Could you check a few things on this model? Use its own coordinates, in mm. Face numbers are marked on the shaded views. A direction names the side the tool comes from. Round coordinates to 2 decimals unless told otherwise and drop trailing zeros. Order: outer loops, then holes, each group sorted by start corner. A loop starts at its lowest first (then second) coordinate and runs counter-clockwise, first axis right, second up. Notation, with made-up numbers: (85, 39.5) - (97, 39.5) arc R6 ccw to (97, 50.5) - close; hole circle Ø4 at (35, 76). An arc over 180 degrees is marked (long way). Return JSON: item names as keys, results as strings. Group by question number.
from build123d import *

# Parameters (mm, degrees)
CROQUIS1_R              = 2.5
SALIENTE_EXTRUIR1_DEPTH = 36.2
CROQUIS2_OUTSIDE_W      = 14.376
CROQUIS2_OUTSIDE_H      = 14.376
CROQUIS2_OUTSIDE_W_2    = 5.186631864
CROQUIS2_OUTSIDE_H_2    = 3
CORTAR_EXTRUIR1_DEPTH   = 8
CROQUIS2_3_R            = 0.79375
CORTAR_EXTRUIR2_DEPTH   = 5
CROQUIS3_OUTSIDE_W      = 14.376
CROQUIS3_OUTSIDE_H      = 14.376
CORTAR_EXTRUIR3_DEPTH   = 8
CROQUIS4_R              = 0.79375
CORTAR_EXTRUIR4_DEPTH   = 5


with BuildPart() as part:
    # Croquis1 → Saliente-Extruir1 (new body)
    with BuildSketch(Plane(origin=(0, 0, 0), x_dir=(0, 0, -1), z_dir=(1, 0, 0))):
        Circle(CROQUIS1_R)
    extrude(amount=SALIENTE_EXTRUIR1_DEPTH)

    # Croquis2 outside → Cortar-Extruir1 (cut)
    with BuildSketch(Plane(origin=(36.2, 0, 0), x_dir=(0, 0, -1), z_dir=(1, 0, 0))):
        Rectangle(CROQUIS2_OUTSIDE_W, CROQUIS2_OUTSIDE_H)
        Rectangle(CROQUIS2_OUTSIDE_W_2, CROQUIS2_OUTSIDE_H_2, mode=Mode.SUBTRACT)
    extrude(amount=-CORTAR_EXTRUIR1_DEPTH, mode=Mode.SUBTRACT)

    # Croquis2_3 → Cortar-Extruir2 (cut)
    with BuildSketch(Plane(origin=(36.2, 0, 0), x_dir=(0, 0, -1), z_dir=(1, 0, 0))):
        Circle(CROQUIS2_3_R)
    extrude(amount=-CORTAR_EXTRUIR2_DEPTH, mode=Mode.SUBTRACT)

    # Croquis3 outside → Cortar-Extruir3 (cut)
    with BuildSketch(Plane(origin=(0, 0, 0), x_dir=(0, 0, -1), z_dir=(1, 0, 0))):
        Rectangle(CROQUIS3_OUTSIDE_W, CROQUIS3_OUTSIDE_H)
        with BuildLine():
            Line((2, 1.5), (-2, 1.5))
            ThreePointArc((-2, 1.5), (-2.5, 0), (-2, -1.5))
            Line((-2, -1.5), (2, -1.5))
            ThreePointArc((2, -1.5), (2.5, 0), (2, 1.5))
        make_face(mode=Mode.SUBTRACT)
    extrude(amount=CORTAR_EXTRUIR3_DEPTH, mode=Mode.SUBTRACT)

    # Croquis4 → Cortar-Extruir4 (cut)
    with BuildSketch(Plane.ZY):
        Circle(CROQUIS4_R)
    extrude(amount=-CORTAR_EXTRUIR4_DEPTH, mode=Mode.SUBTRACT)


solid = part.part
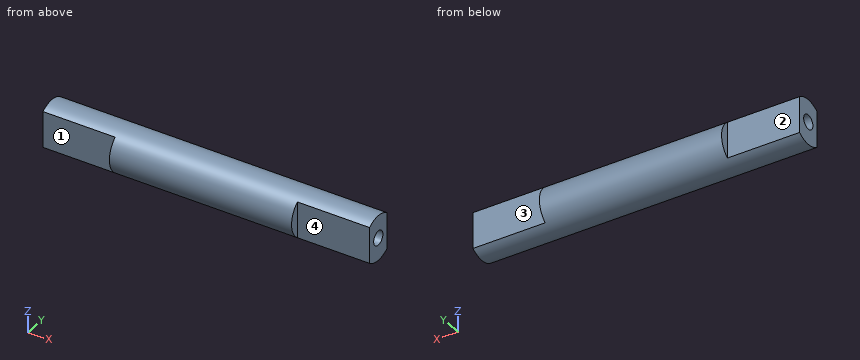
1) I want a section at C-C, the plane z = -1.5. List the corners of the cut face in (x, y) for me.
2) I want a section at D-D, the plane x = 27. List the corners of the cut face in (y, z) for me, plus the area to 3 significant figures.
3) Will these pins go through, and if not, where does the flat tip stop? pin 1 (0.8 mm diameter, centred on y = -2, z = -1, fed in from -X); pin 2 (1.3 mm diameter, centred on y = 0, z = 0, fed in from -X); pin 3 (3 mm diameter, centred on x = 4, z = -1, fed in from -Y).
4) I want a section at A-A, the plane y = 0. List the corners of the cut face in (x, z) for me, plus the area to 3 significant figures.
5) For the marked faces 1, 2, 3 and 4, which set-ups out of +Z, -Z, +X, -X, +Y, -Y let a thin tool reach every point of the face, with its end or its side?
6) If I drill on line 1 along Y through (x, z) = (2.2, 0); line 2 along X through (y, z) = (1.75, 1.75); line 3 along Y through (x, z) = (20, -2), over which ranges is the centre line in solid material (lowest first)? Write a range as from..to.
7) I want a section at B-B, the plane x = 31.5. List the corners of the cut face in (y, z) for me.
Outcome:
{
 "1": {"outline": "(0, -1.5) - (8, -1.5) - (8, -2) - (28.2, -2) - (28.2, -1.5) - (36.2, -1.5) - (36.2, 1.5) - (28.2, 1.5) - (28.2, 2) - (8, 2) - (8, 1.5) - (0, 1.5) - close"},
 "2": {"outline": "circle Ø5 at (0, 0)", "area": "19.6 mm^2"},
 "3": {"pin 1": "x = 8", "pin 2": "x = 5", "pin 3": "y = -1.5"},
 "4": {"outline": "(0, -2.5) - (36.2, -2.5) - (36.2, -0.79) - (31.2, -0.79) - (31.2, 0.79) - (36.2, 0.79) - (36.2, 2.5) - (0, 2.5) - (0, 0.79) - (5, 0.79) - (5, -0.79) - (0, -0.79) - close", "area": "165 mm^2"},
 "5": {"face 1": "+Z, -Z, -X, -Y", "face 2": "+Z, -Z, -X, +Y", "face 3": "+Z, -Z, +X, +Y", "face 4": "+Z, -Z, +X, -Y"},
 "6": {"line 1": "-1.5..-0.79, 0.79..1.5", "line 2": "8..28.2", "line 3": "-1.5..1.5"},
 "7": {"outline": "(-1.5, -2) arc R2.5 ccw to (1.5, -2) - (1.5, 2) arc R2.5 ccw to (-1.5, 2) - close; hole circle Ø1.59 at (0, 0)"}
}
